Job drawing, mm, ordinate dimensions from the low corner. One solid piece. A direction names the side the tool comes from. Give positions to 0.01 mm unless a question says otherwise; leave off trailing zeros. Write each loop counter-clockwise with the first axis right and the second up, starting at its lowest first coordinate (ties: lowest second). Pieces come first, ordered by that corner, then holes. Notation, with made-up numbers: (70, 15.25) - (126, 15.25) arc R17 ccw to (126, 46.25) - close; hole circle Ø6 at (-8.75, -39). An arc over 180 degrees is marked (long way). Answer as a JSON object with one key per item and string values.
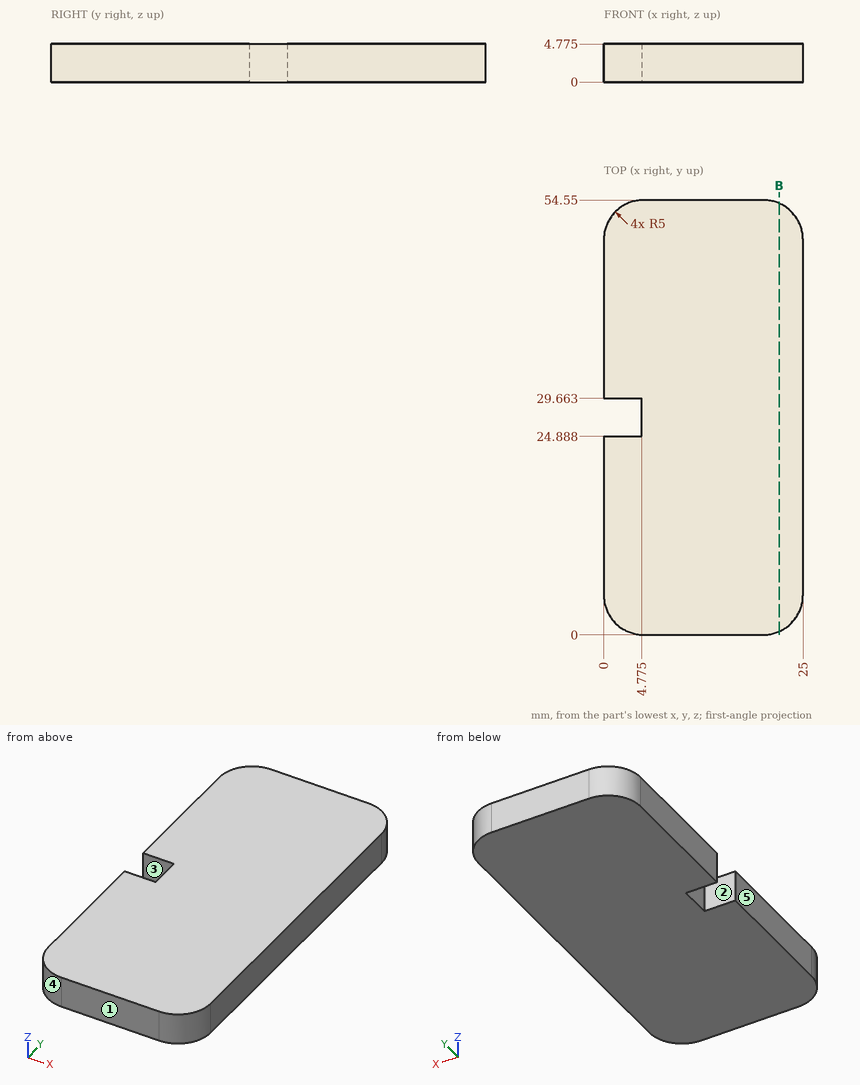
Item 1: Flat gauge pins, fed straight in: P1, Ø1.4, axis at x = 3, z = 1.5, coming from the +Y side; P2, Ø1.4, axis at y = 26, z = 1.5, coming from the -X side (1 decimal). Where does each tip first touch, or does it go through?
Entries:
{"P1": "y = 54.38", "P2": "x = 4.8"}
Item 2: Cut at B-B (x = 22). Give the cut face in (y, z) (1 decimal).
Entries:
{"outline": "(0.4, 0) - (54.1, 0) - (54.1, 4.8) - (0.4, 4.8) - close"}
Item 3: Mould opens along Y. For the marked faces 3, 4 and 5 say: +Y half, -Y half, draft (parallel to the pull), parting line (faces both ways), or undercut.
Entries:
{"face 3": "undercut", "face 4": "-Y half", "face 5": "draft"}
Item 4: Probe line 1 (X direction, y = 27, z = 2.85) (1 decimal); line 2 (Y direction, x = 1.25, z = 1.7) (1 decimal); line 3 (Y direction, x = 22.5, z = 2.05). List the from-to ranges inside material, lowest first. Write a range as from..to.
Entries:
{"line 1": "4.8..25", "line 2": "1.7..24.9, 29.7..52.9", "line 3": "0.67..53.88"}
Item 5: Which spindle directions (+Z, -Z, +X, -X, +Y, -Y) get a long thin tool onto all of the face, cutting with end or side? Do the marked faces 1 and 2. Say none if no direction does.
Entries:
{"face 1": "+Z, -Z, +X, -X, -Y", "face 2": "+Z, -Z, -X"}
